```python
from build123d import *

# Parameters (mm, degrees)
SKETCH_1_W          = 70
SKETCH_1_H          = 60
SKETCH_1_R          = 2.5
EXTRUDE_1_DEPTH     = 5
EXTRUDE_2_DEPTH     = 70
CUT_EXTRUDE_1_DEPTH = 70
SKETCH_4_R          = 2.5
CUT_EXTRUDE_2_DEPTH = 5


with BuildPart() as part:
    # 草图1 → 凸台-拉伸1 (new body)
    with BuildSketch(Plane.XY):
        Rectangle(SKETCH_1_W, SKETCH_1_H)
        with Locations((-20, 15)):
            Circle(SKETCH_1_R, mode=Mode.SUBTRACT)
        with Locations((20, 15)):
            Circle(SKETCH_1_R, mode=Mode.SUBTRACT)
        with Locations((-20, -15)):
            Circle(SKETCH_1_R, mode=Mode.SUBTRACT)
        with Locations((20, -15)):
            Circle(SKETCH_1_R, mode=Mode.SUBTRACT)
    extrude(amount=EXTRUDE_1_DEPTH)

    # 草图2 → 凸台-拉伸2 (add)
    with BuildSketch(Plane.XY.offset(5)):
        Polygon((-30, 30), (-35, 30), (-35, -30), (35, -30), (35, 30), (30, 30), (30, -25), (-30, -25), align=None)
    extrude(amount=EXTRUDE_2_DEPTH)

    # 草图3 → 切除-拉伸1 (cut)
    with BuildSketch(Plane.ZY.offset(35)):
        Polygon((5, 30), (75, -25), (75, 30), align=None)
    extrude(amount=-CUT_EXTRUDE_1_DEPTH, mode=Mode.SUBTRACT)

    # 草图4 → 切除-拉伸2 (cut)
    with BuildSketch(Plane.XZ.offset(30)):
        with Locations(Location((-20, 65, 0), (0, 0, 270))):
            Circle(SKETCH_4_R)
        with Locations(Location((20, 65, 0), (0, 0, 270))):
            Circle(SKETCH_4_R)
        with Locations(Location((-20, 45, 0), (0, 0, 270))):
            Circle(SKETCH_4_R)
        with Locations(Location((20, 45, 0), (0, 0, 270))):
            Circle(SKETCH_4_R)
    extrude(amount=-CUT_EXTRUDE_2_DEPTH, mode=Mode.SUBTRACT)


solid = part.part
```
Work out the finished part from the listing and answer in its coordinate system (mm). A direction names the side the tool comes from. Give positions to 0.01 mm unless a question says otherwise; leave off trailing zeros. Write each loop counter-clockwise with the first axis right and the second up, starting at its lowest first coordinate (ties: lowest second). Pieces come first, ordered by that corner, then holes. Notation, with made-up numbers: (0, 34.5) - (32, 34.5) arc R18 cw to (32, 47.5) - close; hole circle Ø9 at (-23, -10.75). An arc over 180 degrees is marked (long way). Use one line per item in the form item = value.
1. Each of these flat-tipped pins is pushed along its axis until it touches: pin 1 Ø4 at (x, z) = (-18, 66) entering from +Y; pin 2 Ø4.5 at (x, y) = (-20, 15) entering from -Z; pin 3 Ø8 at (x, y) = (20, 15) entering from +Z. Where does it stop, or does it pass through?
Filled in:
pin_1 = -25
pin_2 = through
pin_3 = 5
2. A cutting plane is placed at A-A (x = -20). Write down the section's boundary in (y, z), and give its area (3 significant figures).
Filled in:
outline = (-30, 0) - (-17.5, 0) - (-17.5, 5) - (-25, 5) - (-25, 42.5) - (-30, 42.5) - close; (-30, 47.5) - (-25, 47.5) - (-25, 62.5) - (-30, 62.5) - close; (-30, 67.5) - (-25, 67.5) - (-25, 75) - (-30, 75) - close; (-12.5, 0) - (12.5, 0) - (12.5, 5) - (-12.5, 5) - close; (17.5, 0) - (30, 0) - (30, 5) - (17.5, 5) - close
area = 550 mm^2
3. For faces 1 (the face through (0, -27, 75)), 2 (the face through (30, -9, 24)), determine the directions among +Z, -Z, +X, -X, +Y, -Y from which every point of the face is accessible in a straight line to the end or side of a thin tool.
Filled in:
face_1 = +Z, +X, -X, +Y, -Y
face_2 = +Z, +Y
4. A cutting plane is placed at D-D (x = -2). Write down the section's boundary in (y, z).
Filled in:
outline = (-30, 0) - (30, 0) - (30, 5) - (-25, 5) - (-25, 75) - (-30, 75) - close
5. Determine the mould class of faces 3 (the face through (-32.535, 2.885, 39.51)), 4 (the face through (22.11, -27.54, 43.66)), 5 (the face through (0, 30, 2)), 6 (the face through (-19.249, -27.535, 62.615)) for opening direction Z: released by +Z, released by -Z, zero draft, split by the parting line, or undercut.
Filled in:
face_3 = released by +Z
face_4 = undercut
face_5 = zero draft
face_6 = undercut
6. Consider L1, parallel to Y at x = 20, z = 2.1; L2, parallel to X at y = -28.4, z = 45; L3, parallel to X at y = -20, z = 32.5. Determine where each line is inside the solid, lowest interval first.
Filled in:
L1 = -30 to -17.5, -12.5 to 12.5, 17.5 to 30
L2 = -35 to -22.5, -17.5 to 17.5, 22.5 to 35
L3 = -35 to -30, 30 to 35
7. A cutting plane is placed at B-B (y = 15). Write down the section's boundary in (x, z).
Filled in:
outline = (-35, 0) - (-22.5, 0) - (-22.5, 5) - (-30, 5) - (-30, 24.09) - (-35, 24.09) - close; (-17.5, 0) - (17.5, 0) - (17.5, 5) - (-17.5, 5) - close; (22.5, 0) - (35, 0) - (35, 24.09) - (30, 24.09) - (30, 5) - (22.5, 5) - close
8. A cutting plane is placed at C-C (z = 54). Write down the section's boundary in (x, y), and give its area (3 significant figures).
Filled in:
outline = (-35, -30) - (35, -30) - (35, -8.5) - (30, -8.5) - (30, -25) - (-30, -25) - (-30, -8.5) - (-35, -8.5) - close
area = 515 mm^2
